Part model, mm, in its own coordinate system. A direction names the side the tool comes from. Give positions to 0.01 mm unless a question says otherwise; leave off trailing zeros. Order: outer loops, then holes, each group sorted by start corner. A loop starts at its lowest first (then second) coordinate and runs counter-clockwise, first axis right, second up. Notation, with made-up numbers: M -26,31.5 L 31,31.5 A18 ccw 31,57.5 Z; hole C -6,78 d2. An arc over 180 degrees is marked long. One line per question, with ' | ' between items.
```python
from build123d import *

# Parameters (mm, degrees)
SKETCH1_R                 = 1.999996
BOSS_EXTRUDE1_DEPTH       = 6.35
BOSS_EXTRUDE1_2_DEPTH     = 6.35
SKETCH1_3_W               = 34.08
SKETCH1_3_H               = 15.48
BOSS_EXTRUDE2_DEPTH       = 62.5
SKETCH2_W                 = 34.08
SKETCH2_H                 = 15.48
SKETCH2_W_2               = 29
SKETCH2_H_2               = 10.4
BOSS_EXTRUDE3_DEPTH       = 19.4
SKETCH3_W                 = 11.67
SKETCH3_H                 = 21.9
CUT_EXTRUDE1_DEPTH        = 13
SKETCH4_W                 = 5
SKETCH4_H                 = 10.4
BOSS_EXTRUDE4_DEPTH       = 3.2
CUT_EXTRUDE3_DEPTH        = 97.065834197
CUT_EXTRUDE3_DEPTH_BACK   = 97.065834197
F_3_0MM_DOWEL_HOLE1_D     = 3.2
F_3_0MM_DOWEL_HOLE1_DEPTH = 15.48
F_3_0MM_DOWEL_HOLE1_TIP   = 0.96137699
SKETCH10_W                = 13.54
SKETCH10_H                = 10.4
CUT_EXTRUDE5_DEPTH        = 2.5
FILLET1_R                 = 10
CUT_EXTRUDE6_DEPTH        = 53.65
BOSS_EXTRUDE5_DEPTH       = 26.54
FILLET3_R                 = 1


with BuildPart() as part:
    # Sketch1 → Boss-Extrude1 (new body)
    with BuildSketch(Plane(origin=(0, 0, 0), x_dir=(1, 0, 0), z_dir=(0, 1, 0))):
        with BuildLine():
            ThreePointArc((-17.04, 36.95), (-16.296051224, 38.746051224), (-14.5, 39.49))
            Line((-14.5, 39.49), (14.5, 39.49))
            ThreePointArc((14.5, 39.49), (16.296051224, 38.746051224), (17.04, 36.95))
            Line((17.04, 36.95), (17.04, 7.74))
            Line((17.04, 7.74), (-17.04, 7.74))
            Line((-17.04, 7.74), (-17.04, 36.95))
        make_face()
        with Locations(Location((-0.022, 35.68, 0), (0, 0, 270))):
            Circle(SKETCH1_R, mode=Mode.SUBTRACT)
    extrude(amount=BOSS_EXTRUDE1_DEPTH)



with BuildPart() as body_2:
    # Sketch1 → Boss-Extrude1 2 (new body)
    with BuildSketch(Plane(origin=(0, 0, 0), x_dir=(1, 0, 0), z_dir=(0, 1, 0))):
        with BuildLine():
            Line((-17.04, -7.74), (-17.04, -36.95))
            ThreePointArc((-17.04, -36.95), (-16.296051224, -38.746051224), (-14.5, -39.49))
            Line((-14.5, -39.49), (14.5, -39.49))
            ThreePointArc((14.5, -39.49), (16.296051224, -38.746051224), (17.04, -36.95))
            Line((17.04, -36.95), (17.04, -7.74))
            Line((17.04, -7.74), (-17.04, -7.74))
        make_face()
        with Locations(Location((-0.022, -35.68, 0), (0, 0, 270))):
            Circle(SKETCH1_R, mode=Mode.SUBTRACT)
    extrude(amount=BOSS_EXTRUDE1_2_DEPTH)


with BuildPart() as part_1:
    add(part.part)

    add(body_2.part)  # Boss-Extrude2 merges body 2
    # Sketch1<3> → Boss-Extrude2 (add)
    with BuildSketch(Plane(origin=(0, 0, 0), x_dir=(1, 0, 0), z_dir=(0, 1, 0))):
        Rectangle(SKETCH1_3_W, SKETCH1_3_H)
    extrude(amount=BOSS_EXTRUDE2_DEPTH)

    # Sketch2 → Boss-Extrude3 (add)
    with BuildSketch(Plane(origin=(0, 62.5, 0), x_dir=(1, 0, 0), z_dir=(0, 1, 0))):
        Rectangle(SKETCH2_W, SKETCH2_H)
        Rectangle(SKETCH2_W_2, SKETCH2_H_2, mode=Mode.SUBTRACT)
    extrude(amount=BOSS_EXTRUDE3_DEPTH)

    # Sketch3 → Cut-Extrude1 (cut)
    with BuildSketch(Plane(origin=(17.04, 0, 0), x_dir=(0, 0, -1), z_dir=(1, 0, 0))):
        with Locations((0, 70.95)):
            Rectangle(SKETCH3_W, SKETCH3_H)
    extrude(amount=-CUT_EXTRUDE1_DEPTH, mode=Mode.SUBTRACT)

    # Sketch4 → Boss-Extrude4 (add)
    with BuildSketch(Plane(origin=(0, 62.5, 0), x_dir=(1, 0, 0), z_dir=(0, 1, 0))):
        with Locations((-12, 0)):
            Rectangle(SKETCH4_W, SKETCH4_H)
    extrude(amount=BOSS_EXTRUDE4_DEPTH)

    # Sketch5 → Cut-Extrude3 (cut, two sides: drawn at the far end of the back side and taken through both)
    with BuildSketch(Plane(origin=(0, 0, -7.74), x_dir=(-1, 0, 0), z_dir=(0, 0, -1)).offset(-CUT_EXTRUDE3_DEPTH_BACK)):
        with BuildLine():
            Line((-17.04, 81.9), (-17.04, 74.28))
            ThreePointArc((-17.04, 74.28), (-14.808153673, 79.668153673), (-9.42, 81.9))
            Line((-9.42, 81.9), (-17.04, 81.9))
        make_face()
    extrude(amount=CUT_EXTRUDE3_DEPTH + CUT_EXTRUDE3_DEPTH_BACK, mode=Mode.SUBTRACT)

    # Ø3.0mm Dowel Hole1
    with Locations(Plane(origin=(0, 0, -7.74), x_dir=(-1, 0, 0), z_dir=(0, 0, -1))):
        with Locations((11.650000349, 68.85), (-10.400000349, 79.2)):
            Hole(F_3_0MM_DOWEL_HOLE1_D / 2, depth=F_3_0MM_DOWEL_HOLE1_DEPTH)
            with Locations((0, 0, -(F_3_0MM_DOWEL_HOLE1_DEPTH + F_3_0MM_DOWEL_HOLE1_TIP / 2))):  # 118° drill point
                Cone(0, F_3_0MM_DOWEL_HOLE1_D / 2, F_3_0MM_DOWEL_HOLE1_TIP, mode=Mode.SUBTRACT)

    # Sketch10 → Cut-Extrude5 (cut)
    with BuildSketch(Plane(origin=(0, 62.5, 0), x_dir=(1, 0, 0), z_dir=(0, 1, 0))):
        with Locations((-2.73, 0)):
            Rectangle(SKETCH10_W, SKETCH10_H)
    extrude(amount=-CUT_EXTRUDE5_DEPTH, mode=Mode.SUBTRACT)

    # Fillet1
    fillet1_edges = [part_1.edges().sort_by_distance(p)[0] for p in [
        (0, 6.35, -7.74),
        (0, 6.35, 7.74),
    ]]
    fillet(fillet1_edges, radius=FILLET1_R)

    # Sketch11 → Cut-Extrude6 (cut)
    with BuildSketch(Plane(origin=(0, 60, 0), x_dir=(1, 0, 0), z_dir=(0, 1, 0))):
        Polygon((17.04, -5.835), (17.04, 5.835), (4.04, 5.835), (4.04, 5.2), (-9.5, 5.2), (-9.5, -5.2), (4.04, -5.2), (4.04, -5.835), align=None)
    extrude(amount=-CUT_EXTRUDE6_DEPTH, mode=Mode.SUBTRACT)

    # Sketch12 → Boss-Extrude5 (add)
    with BuildSketch(Plane(origin=(-9.5, 0, 0), x_dir=(0, 0, -1), z_dir=(1, 0, 0))):
        Polygon((-5.2, 31.35), (-5.835, 31.35), (-5.835, 6.35), (0, 6.35), (5.835, 6.35), (5.835, 31.35), (5.2, 31.35), (0, 6.45), align=None)
    extrude(amount=BOSS_EXTRUDE5_DEPTH)

    # Fillet3
    fillet3_edges = [part_1.edges().sort_by_distance(p)[0] for p in [
        (3.77, 6.45, 0),
    ]]
    fillet(fillet3_edges, radius=FILLET3_R)


solid = part_1.part
```
1. Slice it at C-C on x = -11.65. Give the cut face in (y, z).
Worked out:
outline: M 0,-39.49 L 6.35,-39.49 L 6.35,-17.74 A10 cw 16.35,-7.74 L 67.25,-7.74 L 67.25,-5.2 L 65.7,-5.2 L 65.7,5.2 L 67.25,5.2 L 67.25,7.74 L 16.35,7.74 A10 cw 6.35,17.74 L 6.35,39.49 L 0,39.49 Z; M 70.45,-7.74 L 81.9,-7.74 L 81.9,-5.2 L 70.45,-5.2 Z; M 70.45,5.2 L 81.9,5.2 L 81.9,7.74 L 70.45,7.74 Z
2. Slice it at D-D on x = -3. Give the cut face in (y, z), then the cut area to 3 significant figures.
Worked out:
outline: M 0,-39.49 L 6.35,-39.49 L 6.35,-17.74 A10 cw 16.35,-7.74 L 81.9,-7.74 L 81.9,-5.2 L 31.35,-5.2 L 11.14,-0.98 A1 cw 11.14,0.98 L 31.35,5.2 L 81.9,5.2 L 81.9,7.74 L 16.35,7.74 A10 cw 6.35,17.74 L 6.35,39.49 L 0,39.49 Z | area: 1,060 mm2
3. Slice it at B-B on z = 35.68. Give the cut face in (x, y), then the cut area to 3 significant figures.
Worked out:
outline: M -17.04,0 L -2.02,0 L -2.02,6.35 L -17.04,6.35 Z; M 1.98,0 L 17.04,0 L 17.04,6.35 L 1.98,6.35 Z | area: 191 mm2
4. Slice it at A-A on y = 68.85. Give the cut face in (x, z) (3 decimals).
Worked out:
outline: M -17.04,-7.74 L -13.25,-7.74 L -13.25,-5.2 L -14.5,-5.2 L -14.5,5.2 L -13.25,5.2 L -13.25,7.74 L -17.04,7.74 Z; M -10.05,-7.74 L 17.04,-7.74 L 17.04,-5.835 L 4.04,-5.835 L 4.04,-5.2 L -10.05,-5.2 Z; M -10.05,5.2 L 4.04,5.2 L 4.04,5.835 L 17.04,5.835 L 17.04,7.74 L -10.05,7.74 Z
5. Probe L1, parallel to Z at x = -10, y = 73.5; L2, parallel to Z at x = 5.5, y = 74.5 (3 decimals); L3, parallel to X at y = 5, z = 35.68. List the from-to ranges inside material, lowest first. Write a range as from..to.
Worked out:
L1: z = -7.74..-5.2, 5.2..7.74 | L2: z = -7.74..-5.835, 5.835..7.74 | L3: x = -17.04..-2.02, 1.98..17.04
6. Mould opens along Y. For faces 1 (the flat face through (-12, 65.7, 0)), 2 (the cylindrical face through (11.26, 80.55, 6.8)), 3 (the flat face through (-14.5, 74, 0)) say: released by +Y, released by -Y, zero draft, split by the parting line, or undercut.
Worked out:
face 1: released by +Y | face 2: undercut | face 3: zero draft
7. Drop flat-ended pins along their axis: pin 1 (0.5 mm diameter, centred on y = 44.5, z = -5.5, fed in from +X); pin 2 (14.5 mm diameter, centred on x = 11, y = 50.5, fed in from -Z); pin 3 (12 mm diameter, centred on y = 62, z = -11, fed in from -X); pin 4 (11 mm diameter, centred on x = 3, z = -23.5, fed in from +Y). Give the stop position or say it passes through.
Worked out:
pin 1: stops at x = 4.04 | pin 2: stops at z = -7.74 | pin 3: stops at x = -17.04 | pin 4: stops at y = 6.35
8. Tool access for faces 4 (the flat face through (0, 49, -7.74)), 5 (the flat face through (11, 56, 5.835)), 6 (the cylindrical face through (14.867, 79.609, 6.801)), 7 (the cylindrical face through (-16, 3, -39)), 8 (the flat face through (0, 49, 7.74)): list every direction of +Z, -Z, +X, -X, +Y, -Y with a clear straight run to the whole face (end or side of a thin tool).
Worked out:
face 4: -Z, +X, -X, +Y | face 5: +X, +Y | face 6: +Z, -Z, +X, +Y | face 7: -Z, -X, +Y, -Y | face 8: +Z, +X, -X, +Y
